from build123d import *

# Parameters (mm, degrees)
F0_R     = 1.5
F0_R_2   = 10
F1_DEPTH = 3
F2_DEPTH = 33
F3_DEPTH = 20


with BuildPart() as f1:
    # F0 (on Top) → F1 (new body)
    with BuildSketch(Plane.XY):
        with BuildLine():
            Line((-12.9903810568, -7.5), (-10.8253175473, -6.25))
            ThreePointArc((-10.8253175473, -6.25), (-2.1706022208, -12.3100969127), (8.0348451211, -9.575555539))
            Line((8.0348451211, -9.575555539), (9.6418141453, -11.4906666468))
            ThreePointArc((9.6418141453, -11.4906666468), (11.4906666468, -9.6418141453), (12.9903810568, -7.5))
            Line((12.9903810568, -7.5), (10.8253175473, -6.25))
            ThreePointArc((10.8253175473, -6.25), (11.7461577598, 4.2752517916), (4.2752517916, 11.7461577598))
            Line((4.2752517916, 11.7461577598), (5.1303021499, 14.0953893118))
            ThreePointArc((5.1303021499, 14.0953893118), (2.604722665, 14.7721162952), (0, 15))
            Line((0, 15), (0, 12.5))
            ThreePointArc((0, 12.5), (-9.575555539, 8.0348451211), (-12.3100969127, -2.1706022208))
            Line((-12.3100969127, -2.1706022208), (-14.7721162952, -2.604722665))
            ThreePointArc((-14.7721162952, -2.604722665), (-14.0953893118, -5.1303021499), (-12.9903810568, -7.5))
        make_face()
        with Locations((-11.7461577598, -4.2752517916)):
            Circle(F0_R, mode=Mode.SUBTRACT)
        with Locations((9.575555539, -8.0348451211)):
            Circle(F0_R, mode=Mode.SUBTRACT)
        Circle(F0_R_2, mode=Mode.SUBTRACT)
        with Locations((2.1706022208, 12.3100969127)):
            Circle(F0_R, mode=Mode.SUBTRACT)
        Circle(F0_R_2)
        with BuildLine():
            ThreePointArc((1.1180339887, 1), (0, -1.5), (-1.1180339887, 1))
            Line((-1.1180339887, 1), (1.1180339887, 1))
        make_face(mode=Mode.SUBTRACT)
    extrude(amount=F1_DEPTH)

    # F0 (on Top) → F2 (join)
    with BuildSketch(Plane.XY):
        with BuildLine():
            Line((-12.9903810568, -7.5), (-10.8253175473, -6.25))
            ThreePointArc((-10.8253175473, -6.25), (-2.1706022208, -12.3100969127), (8.0348451211, -9.575555539))
            Line((8.0348451211, -9.575555539), (9.6418141453, -11.4906666468))
            ThreePointArc((9.6418141453, -11.4906666468), (11.4906666468, -9.6418141453), (12.9903810568, -7.5))
            Line((12.9903810568, -7.5), (10.8253175473, -6.25))
            ThreePointArc((10.8253175473, -6.25), (11.7461577598, 4.2752517916), (4.2752517916, 11.7461577598))
            Line((4.2752517916, 11.7461577598), (5.1303021499, 14.0953893118))
            ThreePointArc((5.1303021499, 14.0953893118), (2.604722665, 14.7721162952), (0, 15))
            Line((0, 15), (0, 12.5))
            ThreePointArc((0, 12.5), (-9.575555539, 8.0348451211), (-12.3100969127, -2.1706022208))
            Line((-12.3100969127, -2.1706022208), (-14.7721162952, -2.604722665))
            ThreePointArc((-14.7721162952, -2.604722665), (-14.0953893118, -5.1303021499), (-12.9903810568, -7.5))
        make_face()
        with Locations((-11.7461577598, -4.2752517916)):
            Circle(F0_R, mode=Mode.SUBTRACT)
        with Locations((9.575555539, -8.0348451211)):
            Circle(F0_R, mode=Mode.SUBTRACT)
        Circle(F0_R_2, mode=Mode.SUBTRACT)
        with Locations((2.1706022208, 12.3100969127)):
            Circle(F0_R, mode=Mode.SUBTRACT)
    extrude(amount=F2_DEPTH)

    # F0 (on Top) → F3 (join)
    with BuildSketch(Plane.XY):
        with BuildLine():
            Line((1.1180339887, 1), (-1.1180339887, 1))
            ThreePointArc((-1.1180339887, 1), (0, -1.5), (1.1180339887, 1))
        make_face()
    extrude(amount=F3_DEPTH)


solid = f1.part
Could you check a few things on this model? Use its own coordinates, in mm. A direction names the side the tool comes from. Give positions to 0.01 mm unless a question says otherwise; leave off trailing zeros. Order: outer loops, then holes, each group sorted by start corner. A loop starts at its lowest first (then second) coordinate and runs counter-clockwise, first axis right, second up. Notation, with made-up numbers: (38.5, 7.25) -> (95.5, 7.25) arc R36 cw to (95.5, 43.25) -> close; hole circle Ø10 at (88.25, -7). An arc over 180 degrees is marked (long way). Return JSON: item names as keys, results as strings.
1. Imagine slicing it at C-C on z = 20.5. List the corners of the cut face in (x, y) for me, then the cut area to 3 significant figures.
Answer list:
{"outline": "(-14.77, -2.6) arc R15 ccw to (-12.99, -7.5) -> (-10.83, -6.25) arc R12.5 ccw to (8.03, -9.58) -> (9.64, -11.49) arc R15 ccw to (12.99, -7.5) -> (10.83, -6.25) arc R12.5 ccw to (4.28, 11.75) -> (5.13, 14.1) arc R15 ccw to (0, 15) -> (0, 12.5) arc R12.5 ccw to (-12.31, -2.17) -> close; hole circle Ø3 at (-11.75, -4.28); hole circle Ø20 at (0, 0); hole circle Ø3 at (2.17, 12.31); hole circle Ø3 at (9.58, -8.03)", "area": "192 mm2"}
2. I need wall thicknesses on line 1 (X direction, y = 0, z = 26); line 2 (X direction, y = -0.5, z = 9.5); line 3 (X direction, y = -8.25, z = 4). Which ranges of each line are inside material? Lowest first, please. Write a range as from..to.
Answer list:
{"line 1": "x = -12.5..-10, 10..12.5", "line 2": "x = -12.49..-9.99, -1.41..1.41, 9.99..12.49", "line 3": "x = -9.39..-5.65, 5.65..8.09, 11.06..12.53"}
3. Imagine slicing it at D-D on x = -9.5. List the corners of the cut face in (y, z) for me, then the cut area to 3 significant figures.
Answer list:
{"outline": "(-8.12, 0) -> (8.12, 0) -> (8.12, 33) -> (3.12, 33) -> (3.12, 3) -> (-3.12, 3) -> (-3.12, 33) -> (-8.12, 33) -> close", "area": "349 mm2"}
4. Imagine slicing it at A-A on y = 0. List the corners of the cut face in (x, z) for me, then the cut area to 3 significant figures.
Answer list:
{"outline": "(-12.5, 0) -> (12.5, 0) -> (12.5, 33) -> (10, 33) -> (10, 3) -> (1.5, 3) -> (1.5, 20) -> (-1.5, 20) -> (-1.5, 3) -> (-10, 3) -> (-10, 33) -> (-12.5, 33) -> close", "area": "276 mm2"}
5. Thinking about a two-plate mould opening in X: for faces 5 (the flat face through (-13.524, -2.385, 16.269)), 6 (the cylindrical face through (-11.941, -2.788, 16.269)), 7 (the cylindrical face through (11.8, 4.13, 16.27)), 8 (the flat face through (-1, -2, 0)), which applies, pulls with the +X half, pulls with the -X half, needs draft (parallel to the pull), parting line crosses it, or undercut?
Answer list:
{"face 5": "pulls with the -X half", "face 6": "undercut", "face 7": "pulls with the +X half", "face 8": "needs draft"}
6. On a 3-axis mill with a long thin cutter (end or side, diameter ignored), from which of +Z, -Z, +X, -X, +Y, -Y can I reach the whole of each face in a straight line? I mean faces 1 (the flat face through (4.697, 12.904, 16.269)), 2 (the flat face through (0, 14, 16)), 3 (the cylindrical face through (11.467, -9.67, 16.269)), 4 (the cylindrical face through (-2.17, -9.76, 17.79)). Say none if no direction works.
Answer list:
{"face 1": "+Z, -Z, +X", "face 2": "+Z, -Z, -X, +Y", "face 3": "+Z, -Z, +X, -Y", "face 4": "+Z"}
7. Imagine slicing it at B-B on z = 11. List the corners of the cut face in (x, y) for me, then the cut area to 3 significant figures.
Answer list:
{"outline": "(-14.77, -2.6) arc R15 ccw to (-12.99, -7.5) -> (-10.83, -6.25) arc R12.5 ccw to (8.03, -9.58) -> (9.64, -11.49) arc R15 ccw to (12.99, -7.5) -> (10.83, -6.25) arc R12.5 ccw to (4.28, 11.75) -> (5.13, 14.1) arc R15 ccw to (0, 15) -> (0, 12.5) arc R12.5 ccw to (-12.31, -2.17) -> close; (-1.12, 1) arc R1.5 ccw (long way) to (1.12, 1) -> close; hole circle Ø3 at (-11.75, -4.28); hole circle Ø20 at (0, 0); hole circle Ø3 at (2.17, 12.31); hole circle Ø3 at (9.58, -8.03)", "area": "198 mm2"}
8. For pin 1 Ø1.5 at (x, z) = (-5, 19) entering from -Y; pin 2 Ø3 at (y, z) = (-8, 19.5) entering from -X; pin 3 Ø1 at (x, z) = (-2.5, 18.5) entering from -Y, each with a flat end and sliding along its axis, tell me the tip position at first contact or that it passes through.
Answer list:
{"pin 1": "stops at y = -11.76", "pin 2": "stops at x = -13.52", "pin 3": "stops at y = -12.34"}
